Can you work these out from the model? Positions are in its coordinate system, mm. A direction names the side the tool comes from. Coordinates: 2 decimals unless noted, no trailing zeros. Order: outer loops, then holes, each group sorted by start corner. A loop starts at its lowest first (then second) coordinate and runs counter-clockwise, first axis right, second up. Notation, with made-up numbers: (10.25, 21.25) -> (66.25, 21.25) arc R14 cw to (66.25, 28.25) -> close; hole circle Ø1 at (-18.75, -29.75). An arc over 180 degrees is marked (long way). Write item = value, one per line.
```python
from build123d import *

# Parameters (mm, degrees)
SKICA2_R                 = 11.379305307
ODEBRAT_VYSUNUT_M1_DEPTH = 18
SKICA3_R                 = 12.741299312
P_IDAT_VYSUNUT_M1_DEPTH  = 18


with BuildPart() as part:
    # Skica1 → Rotovat1 (revolve)
    with BuildSketch(Plane.XY, mode=Mode.PRIVATE) as rotovat1_sk:
        Polygon((0, 9.5), (0, 13.5), (26, 13.5), (26, 5.75), (30, 5.75), (30, 10), (47, 10), (47, 3), (30.5, 3), (30.5, 2), (23, 2), (23, 3), (20, 3), (20, 9.5), align=None)
    revolve(rotovat1_sk.sketch.rotate(Axis((0, 0, 0), (1, 0, 0)), 90), axis=Axis((0, 0, 0), (1, 0, 0)))

    # Skica2 → Odebrat vysunutím1 (cut)
    with BuildSketch(Plane(origin=(47, 0, 0), x_dir=(0, 0, -1), z_dir=(1, 0, 0))):
        Circle(SKICA2_R)
        Polygon((0, 9.814954576), (-8.5, 4.907477288), (-8.5, -4.907477288), (0, -9.814954576), (8.5, -4.907477288), (8.5, 4.907477288), align=None, mode=Mode.SUBTRACT)
    extrude(amount=-ODEBRAT_VYSUNUT_M1_DEPTH, mode=Mode.SUBTRACT)

    # Skica3 → Přidat vysunutím1 (add)
    with BuildSketch(Plane(origin=(26, 0, 0), x_dir=(0, 0, -1), z_dir=(1, 0, 0))):
        Polygon((0, 15.588457268), (-13.5, 7.794228634), (-13.5, -7.794228634), (0, -15.588457268), (13.5, -7.794228634), (13.5, 7.794228634), align=None)
        Circle(SKICA3_R, mode=Mode.SUBTRACT)
    extrude(amount=-P_IDAT_VYSUNUT_M1_DEPTH)


solid = part.part
```
Item 1: For faces 1 (the flat face through (38.619, -7.396, -4.191)), 2 (the flat face through (23, 2, -1)), 3 (the flat face through (8, 7, -12)), 4 (the flat face through (26, -7, 0)), which set-ups out of +Z, -Z, +X, -X, +Y, -Y let a thin tool reach every point of the face, with its end or its side?
A:
face_1 = -Z, +X, -Y
face_2 = -X
face_3 = -Z, -X, +Y
face_4 = none
Item 2: I want a section at D-D, the plane z = 11. Please give me the cut outline in (x, y).
A:
outline = (0, -7.83) -> (8, -7.83) -> (8, -9.24) -> (26, -9.24) -> (26, 9.24) -> (8, 9.24) -> (8, 7.83) -> (0, 7.83) -> close
Item 3: I'm going to push flat-ended pins straight in: P1, Ø5, axis at x = 29.5, y = 0, coming from the -Z side; P2, Ø1.5, axis at x = 36.5, y = 3.5, coming from the +Z side; P3, Ø6, axis at x = 21, z = -4, coming from the +Y side. Where does each tip first touch, or does it pass through?
A:
P1 = -8.5
P2 = 8.5
P3 = 15.01
Item 4: If I drill on probe 1 along Y at (x, z) = (27.5, 0); probe 2 along Y at (x, z) = (20.85, 0); probe 3 along X at (y, z) = (-8, -3), over which ranges is the centre line in solid material (lowest first)?
A:
probe_1 = -5.75 to -2, 2 to 5.75
probe_2 = -15.59 to -3, 3 to 15.59
probe_3 = 20 to 26, 30 to 47
Item 5: If we mould it in two halves opening along Y, with no side actions, what happens to faces 5 (the flat face through (17.13, 11.64, -6.84)), 6 (the cylindrical face through (21.48, -0.9, 2.86)), 7 (the flat face through (39, 0, -8.5))? For each: pulls with the +Y half, pulls with the -Y half, needs draft (parallel to the pull), parting line crosses it, or undercut.
A:
face_5 = pulls with the +Y half
face_6 = undercut
face_7 = needs draft
Item 6: I want a section at A-A, the plane x = 10. Please give me the cut outline in (y, z), plus the area to 3 significant figures.
A:
outline = (-15.59, 0) -> (-7.79, -13.5) -> (7.79, -13.5) -> (15.59, 0) -> (7.79, 13.5) -> (-7.79, 13.5) -> close; hole circle Ø19 at (0, 0)
area = 348 mm2
Item 7: I want a section at C-C, the plane y = 6.5. Please give me the cut outline in (x, z).
A:
outline = (0, -11.83) -> (8, -11.83) -> (8, -13.5) -> (26, -13.5) -> (26, 13.5) -> (8, 13.5) -> (8, 11.83) -> (0, 11.83) -> (0, 6.93) -> (20, 6.93) -> (20, -6.93) -> (0, -6.93) -> close; (30, -5.74) -> (47, -5.74) -> (47, 5.74) -> (30, 5.74) -> close
